Source: CAD feature listing. Evaluate the final solid. Frame: model axes, mm. Face numbers are marked on the shaded views. A direction names the side the tool comes from. Round coordinates to 2 decimals unless told otherwise and drop trailing zeros. Order: outer loops, then holes, each group sorted by start corner. A loop starts at its lowest first (then second) coordinate and runs counter-clockwise, first axis right, second up. Notation, with made-up numbers: (16.25, 71.5) -> (27.25, 71.5) arc R18 ccw to (27.25, 85.5) -> close; hole circle Ø2 at (-9.5, 8). An arc over 180 degrees is marked (long way). Answer as CSV lines item,"result". Start each with the question number.
(1) Section query C-C (y = -9). Output: boundary loops of the cut face in (x, z) (3 decimals), plus the area to 3 significant figures.
(2) Set-up query: the marked faces 4 and 5. Return all of +Z, -Z, +X, -X, +Y, -Y with unobstructed straight access to the full face (end or side cutting, diameter ignored); none if empty.
(3) Contact query for flat-ended pins moving along their axis: P1, Ø4, axis at x = -50, z = 5, coming from the +Y side; P2, Ø4.5, axis at x = -2.5, y = -62, coming from the +Z side (3 decimals); P3, Ø2, axis at y = -43, z = 5, coming from the -X side; P4, Ø10, axis at x = 1.5, y = -49, coming from the +Z side. Output: stop coordinate, or through.
(4) Pull-direction query (X, two-part tool) for the marked faces 1, 2 and 3; classes: +X half, -X half, draft (parallel to the pull), parting line (faces both ways), or undercut.
(5) Section query A-A (x = 0). Output: boundary loops of the cut face in (y, z) (3 decimals), plus the area to 3 significant figures.
(6) Line query: line 1 along Y through (x, z) = (0, 7.25) (3 decimals); line 2 along Z through (x, y) = (-57, 7.5) (3 decimals); line 3 along Y through (x, z) = (63.5, 7.4) (1 decimal). Output: solid intervals per line, ascending. Write a range as from..to.
(7) Section query D-D (z = 15). Output: boundary loops of the cut face in (x, y), plus the area to 3 significant figures.
(8) Section query B-B (z = 2). Output: boundary loops of the cut face in (x, y).
```python
from build123d import *

# Parameters (mm, degrees)
SKETCH2_R           = 73.406
SKETCH2_R_2         = 57.15
BOSS_EXTRUDE1_DEPTH = 19.05
CUT_EXTRUDE5_DEPTH  = 9.525
SKETCH9_R           = 3.175
CUT_EXTRUDE6_DEPTH  = 9.525
CUT_EXTRUDE7_DEPTH  = 5.588


with BuildPart() as part:
    # Sketch2 → Boss-Extrude1 (new body)
    with BuildSketch(Plane.XY):
        Circle(SKETCH2_R)
        Circle(SKETCH2_R_2, mode=Mode.SUBTRACT)
    extrude(amount=BOSS_EXTRUDE1_DEPTH)

    # Sketch7 → Cut-Extrude5 (cut)
    with BuildSketch(Plane.XY.offset(19.05)):
        with BuildLine():
            Line((-69.546757065, 6.501621467), (-55.530220399, 13.5098898))
            ThreePointArc((-55.530220399, 13.5098898), (-57.15, 0), (-55.530220399, -13.5098898))
            Line((-55.530220399, -13.5098898), (-69.546757065, -6.501621467))
            ThreePointArc((-69.546757065, -6.501621467), (-69.85, 0), (-69.546757065, 6.501621467))
        make_face()
        with BuildLine():
            Line((6.501621467, 69.546757065), (13.5098898, 55.530220399))
            ThreePointArc((13.5098898, 55.530220399), (0, 57.15), (-13.5098898, 55.530220399))
            Line((-13.5098898, 55.530220399), (-6.501621467, 69.546757065))
            ThreePointArc((-6.501621467, 69.546757065), (0, 69.85), (6.501621467, 69.546757065))
        make_face()
        with BuildLine():
            Line((69.546757065, -6.501621467), (55.530220399, -13.5098898))
            ThreePointArc((55.530220399, -13.5098898), (57.15, 0), (55.530220399, 13.5098898))
            Line((55.530220399, 13.5098898), (69.546757065, 6.501621467))
            ThreePointArc((69.546757065, 6.501621467), (69.85, 0), (69.546757065, -6.501621467))
        make_face()
        with BuildLine():
            Line((-6.501621467, -69.546757065), (-13.5098898, -55.530220399))
            ThreePointArc((-13.5098898, -55.530220399), (0, -57.15), (13.5098898, -55.530220399))
            Line((13.5098898, -55.530220399), (6.501621467, -69.546757065))
            ThreePointArc((6.501621467, -69.546757065), (0, -69.85), (-6.501621467, -69.546757065))
        make_face()
    extrude(amount=-CUT_EXTRUDE5_DEPTH, mode=Mode.SUBTRACT)

    # Sketch9 → Cut-Extrude6 (cut)
    with BuildSketch(Plane.XY.offset(9.525)):
        with Locations((-63.5, 0)):
            Circle(SKETCH9_R)
        with Locations((0, 63.5)):
            Circle(SKETCH9_R)
        with Locations((63.5, 0)):
            Circle(SKETCH9_R)
        with Locations((0, -63.5)):
            Circle(SKETCH9_R)
    extrude(amount=-CUT_EXTRUDE6_DEPTH, mode=Mode.SUBTRACT)

    # Sketch10 → Cut-Extrude7 (cut)
    with BuildSketch(Plane(origin=(0, 0, 0), x_dir=(-1, 0, 0), z_dir=(0, 0, -1))):
        Polygon((-6.30581964, 63.5), (-3.15290982, 58.039), (3.15290982, 58.039), (6.30581964, 63.5), (3.15290982, 68.961), (-3.15290982, 68.961), align=None)
        Polygon((-63.5, -6.30581964), (-58.039, -3.15290982), (-58.039, 3.15290982), (-63.5, 6.30581964), (-68.961, 3.15290982), (-68.961, -3.15290982), align=None)
        Polygon((63.5, 6.30581964), (58.039, 3.15290982), (58.039, -3.15290982), (63.5, -6.30581964), (68.961, -3.15290982), (68.961, 3.15290982), align=None)
        Polygon((6.30581964, -63.5), (3.15290982, -58.039), (-3.15290982, -58.039), (-6.30581964, -63.5), (-3.15290982, -68.961), (3.15290982, -68.961), align=None)
    extrude(amount=-CUT_EXTRUDE7_DEPTH, mode=Mode.SUBTRACT)


solid = part.part
```
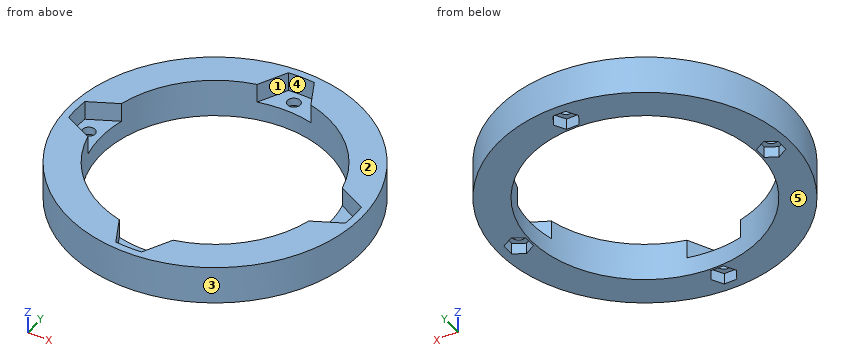
Answer block:
1,outline,"(-72.852, 0) -> (-56.437, 0) -> (-56.437, 9.525) -> (-64.55, 9.525) -> (-64.55, 19.05) -> (-72.852, 19.05) -> close; (56.437, 0) -> (72.852, 0) -> (72.852, 19.05) -> (64.55, 19.05) -> (64.55, 9.525) -> (56.437, 9.525) -> close"
1,area,"471 mm2"
2,face 4,"+Z"
2,face 5,"-Z, +X, -X, +Y, -Y"
3,P1,"y = 55.54"
3,P2,"z = 9.525"
3,P3,"x = -60.2"
3,P4,"through"
4,face 1,"undercut"
4,face 2,"draft"
4,face 3,"parting line"
5,outline,"(-73.406, 0) -> (-68.961, 0) -> (-68.961, 5.588) -> (-66.675, 5.588) -> (-66.675, 9.525) -> (-69.85, 9.525) -> (-69.85, 19.05) -> (-73.406, 19.05) -> close; (-60.325, 5.588) -> (-58.039, 5.588) -> (-58.039, 0) -> (-57.15, 0) -> (-57.15, 9.525) -> (-60.325, 9.525) -> close; (57.15, 0) -> (58.039, 0) -> (58.039, 5.588) -> (60.325, 5.588) -> (60.325, 9.525) -> (57.15, 9.525) -> close; (66.675, 5.588) -> (68.961, 5.588) -> (68.961, 0) -> (73.406, 0) -> (73.406, 19.05) -> (69.85, 19.05) -> (69.85, 9.525) -> (66.675, 9.525) -> close"
5,area,"205 mm2"
6,line 1,"-73.406..-66.675, -60.325..-57.15, 57.15..60.325, 66.675..73.406"
6,line 2,"0..9.525"
6,line 3,"-36.8..-3.2, 3.2..36.8"
7,outline,"circle Ø146.81 at (0, 0); hole (-69.55, -6.5) -> (-55.53, -13.51) arc R57.15 ccw to (-13.51, -55.53) -> (-6.5, -69.55) arc R69.85 ccw to (6.5, -69.55) -> (13.51, -55.53) arc R57.15 ccw to (55.53, -13.51) -> (69.55, -6.5) arc R69.85 ccw to (69.55, 6.5) -> (55.53, 13.51) arc R57.15 ccw to (13.51, 55.53) -> (6.5, 69.55) arc R69.85 ccw to (-6.5, 69.55) -> (-13.51, 55.53) arc R57.15 ccw to (-55.53, 13.51) -> (-69.55, 6.5) arc R69.85 ccw to start"
7,area,"5,650 mm2"
8,outline,"circle Ø146.81 at (0, 0); hole (-68.96, -3.15) -> (-63.5, -6.31) -> (-58.04, -3.15) -> (-58.04, 3.15) -> (-63.5, 6.31) -> (-68.96, 3.15) -> close; hole circle Ø114.3 at (0, 0); hole (-6.31, -63.5) -> (-3.15, -68.96) -> (3.15, -68.96) -> (6.31, -63.5) -> (3.15, -58.04) -> (-3.15, -58.04) -> close; hole (-6.31, 63.5) -> (-3.15, 58.04) -> (3.15, 58.04) -> (6.31, 63.5) -> (3.15, 68.96) -> (-3.15, 68.96) -> close; hole (58.04, -3.15) -> (63.5, -6.31) -> (68.96, -3.15) -> (68.96, 3.15) -> (63.5, 6.31) -> (58.04, 3.15) -> close"
